Build history of the part. All positions in model axes, mm. Round coordinates to 2 decimals unless told otherwise and drop trailing zeros. Write each loop counter-clockwise with the first axis right and the second up, starting at its lowest first coordinate (ties: lowest second). Pieces come first, ordered by that corner, then holes. Notation, with made-up numbers: (-10, 32) -> (8, 32) arc R29 ccw to (8, 53) -> close; hole circle Ø9 at (74, 53). An arc over 180 degrees is marked (long way). One line per question, with ' | ' between items.
from build123d import *

# Parameters (mm, degrees)
F0_W     = 284.226
F0_H     = 190.5
F1_DEPTH = 3.175


with BuildPart() as f1:
    # F0 (on Top) → F1 (new body)
    with BuildSketch(Plane.XY):
        Polygon((307.213, 53.975), (307.213, 155.575), (-307.213, 155.575), (-307.213, -155.575), (-142.113, -155.575), (142.113, -155.575), (307.213, -155.575), (307.213, 34.47796), (291.973, 34.47796), (291.973, 53.975), align=None)
        with Locations((0, -250.825)):
            Rectangle(F0_W, F0_H)
        Polygon((142.113, -346.075), (-142.113, -346.075), (-307.213, -346.075), (-307.213, -657.225), (307.213, -657.225), (307.213, -346.075), align=None)
    extrude(amount=F1_DEPTH)


solid = f1.part
(1) Slice it at B-B (z = 2.4). Write the cut outline in (x, y) (3 decimals), then the cut area to 3 significant figures.
Calculated:
outline: (-307.213, -657.225) -> (307.213, -657.225) -> (307.213, -346.075) -> (142.113, -346.075) -> (142.113, -155.575) -> (307.213, -155.575) -> (307.213, 34.478) -> (291.973, 34.478) -> (291.973, 53.975) -> (307.213, 53.975) -> (307.213, 155.575) -> (-307.213, 155.575) -> (-307.213, -155.575) -> (-142.113, -155.575) -> (-142.113, -346.075) -> (-307.213, -346.075) -> close | area: 436,000 mm2
(2) Slice it at A-A (x = 261). Write the cut outline in (y, z) (3 decimals).
Calculated:
outline: (-657.225, 0) -> (-346.075, 0) -> (-346.075, 3.175) -> (-657.225, 3.175) -> close; (-155.575, 0) -> (155.575, 0) -> (155.575, 3.175) -> (-155.575, 3.175) -> close
(3) Slice it at C-C (y = -207.5). Write the cut outline in (x, z) (3 decimals).
Calculated:
outline: (-142.113, 0) -> (142.113, 0) -> (142.113, 3.175) -> (-142.113, 3.175) -> close
(4) Wall check: line 1 (Y direction, x = 186, z = 0.5) (3 decimals); line 2 (X direction, y = -229, z = 1.5). Give the ranges that are in metal, low to high. Write a range as from..to.
Calculated:
line 1: -657.225..-346.075, -155.575..155.575 | line 2: -142.11..142.11
(5) Drop flat-ended pins along their axis: pin 1 (1.5 mm diameter, centred on x = -85.5, y = -111, fed in from -Z); pin 2 (1 mm diameter, centred on y = -213, z = 1.5, fed in from +X). Give the stop position or say it passes through.
Calculated:
pin 1: z = 0 | pin 2: x = 142.11
